Could you check a few things on this model? Use its own coordinates, in mm. A direction names the side the tool comes from. Give positions to 0.01 mm unless a question says otherwise; leave off trailing zeros. Order: outer loops, then holes, each group sorted by start corner. A loop starts at its lowest first (then second) coordinate and runs counter-clockwise, first axis right, second up.
from build123d import *

# Parameters (mm, degrees)
F0_R     = 4
F1_DEPTH = 10
F2_SIZE  = 0.5
F3_R     = 2.75
F4_DEPTH = 6
F5_R     = 0.5


with BuildPart() as f1:
    # F0 (on Front) → F1 (new body)
    with BuildSketch(Plane.XZ):
        Circle(F0_R)
    extrude(amount=F1_DEPTH)

    # F2
    f2_edges = [f1.edges().sort_by_distance(p)[0] for p in [
        (-4, -10, 0),
    ]]
    chamfer(f2_edges, length=F2_SIZE)

    # F3 (on face) → F4 (cut)
    with BuildSketch(Plane(origin=(0, 0, 0), x_dir=(-1, 0, 0), z_dir=(0, 1, 0))):
        Circle(F3_R)
    extrude(amount=-F4_DEPTH, mode=Mode.SUBTRACT)

    # F5
    f5_edges = [f1.edges().sort_by_distance(p)[0] for p in [
        (-4, 0, 0),
    ]]
    fillet(f5_edges, radius=F5_R)


solid = f1.part
Item 1: Imagine slicing it at C-C on y = -4.5. List the corners of the cut face in (x, z) for me.
Findings:
outline: circle Ø8 at (0, 0); hole circle Ø5.5 at (0, 0)
Item 2: For pin 1 (1.5 mm diameter, centred on y = -3, z = -2, fed in from +X); pin 2 (1.6 mm diameter, centred on x = 0.5, z = -0.5, fed in from +Y), each with a flat end and sliding along its axis, tell me the tip position at first contact or that it passes through.
Findings:
pin 1: stops at x = 3.8
pin 2: stops at y = -6
Item 3: For faces 4 (the flat face through (0, -10, 0)), 5 (the flat face through (0, -6, 0)), which set-ups out of +Z, -Z, +X, -X, +Y, -Y let a thin tool reach every point of the face, with its end or its side?
Findings:
face 4: +Z, -Z, +X, -X, -Y
face 5: +Y
Item 4: Imagine slicing it at B-B on z = 0. List the corners of the cut face in (x, y) for me, then the cut area to 3 significant figures.
Findings:
outline: (-4, -9.5) - (-3.5, -10) - (3.5, -10) - (4, -9.5) - (4, -0.5) arc R0.5 ccw to (3.5, 0) - (2.75, 0) - (2.75, -6) - (-2.75, -6) - (-2.75, 0) - (-3.5, 0) arc R0.5 ccw to (-4, -0.5) - close
area: 46.6 mm2
Item 5: Please list where these lines run through material, in increasing order: line 1 along Z through (x, y) = (0, -2.15); line 2 along Y through (x, z) = (2, 0.75); line 3 along X through (y, z) = (-4.5, -2.25).
Findings:
line 1: z = -4 to -2.75, 2.75 to 4
line 2: y = -10 to -6
line 3: x = -3.31 to -1.58, 1.58 to 3.31
Item 6: We'd pull the mould along Z, two halves only. Please class faces 1 (the flat face through (-3, 0, -1)), 2 (the cylindrical face through (0.596, -2.958, -2.685)), 3 (the cylindrical face through (-0.867, -4.937, -3.905)): +Z half, -Z half, draft (parallel to the pull), parting line (faces both ways), or undercut.
Findings:
face 1: draft
face 2: undercut
face 3: parting line
Item 7: Imagine slicing it at A-A on x = 0. List the corners of the cut face in (y, z) for me.
Findings:
outline: (-10, -3.5) - (-9.5, -4) - (-0.5, -4) arc R0.5 ccw to (0, -3.5) - (0, -2.75) - (-6, -2.75) - (-6, 2.75) - (0, 2.75) - (0, 3.5) arc R0.5 ccw to (-0.5, 4) - (-9.5, 4) - (-10, 3.5) - close
